from build123d import *

# Parameters (mm, degrees)
EXTRUDE_1_DEPTH          = 18
CUT_EXTRUDE_1_DEPTH      = 37
CUT_EXTRUDE_1_DEPTH_BACK = 18
SKETCH_2_R               = 2.5


with BuildPart() as part:
    # 草图1 → 凸台-拉伸1 (new body)
    with BuildSketch(Plane(origin=(0, 0, 0), x_dir=(0, 0, -1), z_dir=(1, 0, 0))):
        Polygon((0, 20), (0, 0), (24, 0), (24, 2), (4, 2), (4, 18), (24, 18), (24, 20), align=None)
    extrude(amount=EXTRUDE_1_DEPTH)

    # 草图2 → 切除-拉伸1 (cut, two sides: drawn at the far end of the back side and taken through both)
    with BuildSketch(Plane(origin=(0, 2, 0), x_dir=(1, 0, 0), z_dir=(0, 1, 0)).offset(-CUT_EXTRUDE_1_DEPTH_BACK)):
        with Locations(Location((9, 16, 0), (0, 0, 90))):
            Circle(SKETCH_2_R)
    extrude(amount=CUT_EXTRUDE_1_DEPTH + CUT_EXTRUDE_1_DEPTH_BACK, mode=Mode.SUBTRACT)


solid = part.part
Design review of the part built by this model. Coordinates are the model's own, in mm. A direction names the side the tool comes from. Give positions to 0.01 mm unless a question says otherwise; leave off trailing zeros. Loops run counter-clockwise (first coordinate to the right, second up) from the corner with the lowest first, then second, coordinate; pieces in that order, holes last. Notation, with made-up numbers: M 11.25,83.25 L 27.25,83.25 A11 ccw 27.25,90.25 Z; hole C 47.25,28.25 d10. An arc over 180 degrees is marked long. Write item = value, one per line.
Q1. For faces 1 (the flat face through (11, 2, -14)), 2 (the flat face through (9, 1, -24)), list the 3-axis set-ups (+Z, -Z, +X, -X, +Y, -Y) from which the entire face can be reached by the end or side of a thin tool; tool diameter is ignored.
Output values:
face_1 = -Z, +X, -X
face_2 = -Z, +X, -X, +Y, -Y
Q2. We need section A-A (x = 9). Give the boundary of the cut face in (y, z), plus the area to 3 significant figures.
Output values:
outline = M 0,-24 L 2,-24 L 2,-18.5 L 0,-18.5 Z; M 0,-13.5 L 2,-13.5 L 2,-4 L 18,-4 L 18,-13.5 L 20,-13.5 L 20,0 L 0,0 Z; M 18,-24 L 20,-24 L 20,-18.5 L 18,-18.5 Z
area = 140 mm^2
Q3. We need section B-B (z = -16). Give the boundary of the cut face in (x, y).
Output values:
outline = M 0,0 L 6.5,0 L 6.5,2 L 0,2 Z; M 0,18 L 6.5,18 L 6.5,20 L 0,20 Z; M 11.5,0 L 18,0 L 18,2 L 11.5,2 Z; M 11.5,18 L 18,18 L 18,20 L 11.5,20 Z
Q4. Insertion check: pin 1 (2 mm diameter, centred on x = 4, y = 9, fed in from -Z); pin 2 (8 mm diameter, centred on y = 13.5, z = -11.5, fed in from -X). Each pin has a flat end and moves straight along its axis. Give the tip position at first contact, or say it passes through.
Output values:
pin_1 = -4
pin_2 = through
Q5. We need section C-C (z = -19.75). Give the boundary of the cut face in (x, y).
Output values:
outline = M 0,0 L 18,0 L 18,2 L 0,2 Z; M 0,18 L 18,18 L 18,20 L 0,20 Z
Q6. Draft analysis for pull direction X (two halves, no side actions). For faces 3 (the flat face through (0, 10.1, -3.8)), 4 (the cylindrical face through (10.5, 1, -14)), 5 (the cylindrical face through (10.5, 19, -14)), 6 (the flat face through (9, 10, 0)), state which applies: +X half, -X half, draft (parallel to the pull), parting line (faces both ways), or undercut.
Output values:
face_3 = -X half
face_4 = undercut
face_5 = undercut
face_6 = draft
Q7. To check wall thickness, follow line 1 (X direction, y = 18.5, z = -16); line 2 (Y direction, x = 4, z = -13.75); line 3 (Z direction, x = 1, y = 16.75). State the ranges of each line that lie inside material, in increasing order. Write a range as [from, to].
Output values:
line_1 = [0, 6.5], [11.5, 18]
line_2 = [0, 2], [18, 20]
line_3 = [-4, 0]
Q8. We need section D-D (y = 1.5). Give the boundary of the cut face in (x, z), plus the area to 3 significant figures.
Output values:
outline = M 0,-24 L 18,-24 L 18,0 L 0,0 Z; hole C 9,-16 d5
area = 412 mm^2
